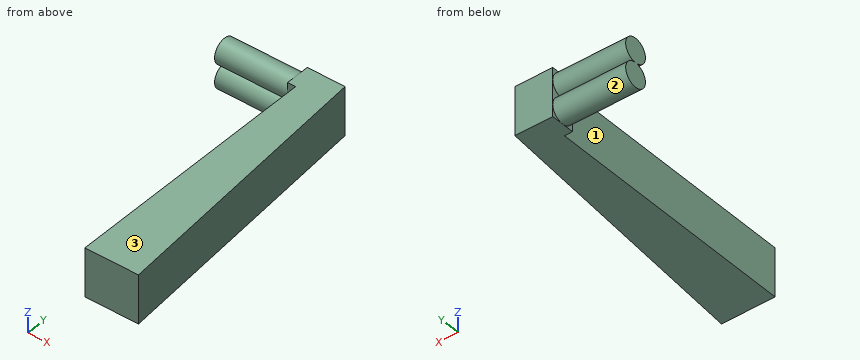
from build123d import *

# Parameters (mm, degrees)
ESTRUSIONE_ESTRUSIONE1_DEPTH      = 30
ESTRUSIONE_ESTRUSIONE1_DEPTH_BACK = 30
ESTRUSIONE_ESTRUSIONE2_DEPTH      = 100
SCHIZZO4_W                        = 60
SCHIZZO4_H                        = 30
ESTRUSIONE_ESTRUSIONE3_DEPTH      = 10


with BuildPart() as part:
    # Schizzo2 → Estrusione-Estrusione1 (new, two sides: drawn at the far end of the back side and taken through both)
    with BuildSketch(Plane.XY.offset(-ESTRUSIONE_ESTRUSIONE1_DEPTH_BACK)):
        Polygon((-15.384222889, 0), (50.78379402, 0), (21.335941259, 350), (-15.384222889, 350), align=None)
    extrude(amount=ESTRUSIONE_ESTRUSIONE1_DEPTH + ESTRUSIONE_ESTRUSIONE1_DEPTH_BACK)

    # Schizzo3 → Estrusione-Estrusione2 (add)
    with BuildSketch(Plane.ZY.offset(15.384222889)):
        with BuildLine():
            Line((-0.032724291, 335.990281697), (0.032724291, 335.990281697))
            ThreePointArc((0.032724291, 335.990281697), (29.999935115, 334.955880248), (0.027157826, 334.097782056))
            Line((0.027157826, 334.097782056), (-0.027157826, 334.097782056))
            ThreePointArc((-0.027157826, 334.097782056), (-29.999935115, 334.955880248), (-0.032724291, 335.990281697))
        make_face()
    extrude(amount=ESTRUSIONE_ESTRUSIONE2_DEPTH)

    # Schizzo4 → Estrusione-Estrusione3 (add)
    with BuildSketch(Plane.ZY.offset(15.384222889)):
        with Locations((0, 335)):
            Rectangle(SCHIZZO4_W, SCHIZZO4_H)
    extrude(amount=ESTRUSIONE_ESTRUSIONE3_DEPTH)


solid = part.part
For this review, take the finished solid that the model builds, in its own axes (mm). Face numbers are marked on the shaded views. Give positions to 0.01 mm unless a question says otherwise; leave off trailing zeros. Write each loop counter-clockwise with the first axis right and the second up, starting at its lowest first coordinate (ties: lowest second). Pieces come first, ordered by that corner, then holes. Notation, with made-up numbers: (23, -2.75) -> (54, -2.75) arc R30 cw to (54, 28.25) -> close; hole circle Ø3 at (-15.75, -34). An arc over 180 degrees is marked (long way). Use CSV: the item, a comma, the result in double quotes.
Q1. For P1, Ø12, axis at y = 210.5, z = -11.5, coming from the -X side; P2, Ø8, axis at x = -19.5, z = -5.5, coming from the -Y side; P3, Ø6, axis at x = -49.5, z = 9.5, coming from the -Y side, all flat-tipped, find the tip position at first contact; note any pin that passes through.
Conclusion:
P1,"x = -15.38"
P2,"y = 320"
P3,"y = 320.21"
Q2. Take a section at C-C, the plane y = 325. Write out the cut boundary in (x, z).
Conclusion:
outline,"(-115.38, -26.18) -> (-25.38, -26.18) -> (-25.38, -30) -> (23.44, -30) -> (23.44, 30) -> (-25.38, 30) -> (-25.38, 26.18) -> (-115.38, 26.18) -> (-115.38, 3.82) -> (-25.38, 3.82) -> (-25.38, -3.82) -> (-115.38, -3.82) -> close"
Q3. Take a section at A-A, the plane z = -23.5. Write out the cut boundary in (x, y), then the cut area to 3 significant figures.
Conclusion:
outline,"(-115.38, 322.64) -> (-25.38, 322.64) -> (-25.38, 320) -> (-15.38, 320) -> (-15.38, 0) -> (50.78, 0) -> (21.34, 350) -> (-25.38, 350) -> (-25.38, 347.36) -> (-115.38, 347.36) -> close"
area,"20,500 mm2"
Q4. Take a section at D-D, the plane y = 240. Write out the cut boundary in (x, z).
Conclusion:
outline,"(-15.38, -30) -> (30.59, -30) -> (30.59, 30) -> (-15.38, 30) -> close"
Q5. To check wall thickness, follow probe 1 along Z at (x, y) = (-41, 330); probe 2 along Y at (x, z) = (-66.5, 14.5); probe 3 along X at (y, z) = (183.5, 4.5). State the ranges of each line that lie inside material, in increasing order. Write a range as [from, to].
Conclusion:
probe 1,"[-29.14, -0.86], [0.86, 29.14]"
probe 2,"[320.01, 349.99]"
probe 3,"[-15.38, 35.34]"
Q6. Take a section at B-B, the plane x = -92. Write out the cut boundary in (y, z).
Conclusion:
outline,"(334.1, -0.03) arc R15 ccw (long way) to (335.99, -0.03) -> (335.99, 0.03) arc R15 ccw (long way) to (334.1, 0.03) -> close"
Q7. Mouldability with a two-part tool opening along Z and no side actions: class the marked faces 1, 2 and 3 as pulls with the +Z half, pulls with the -Z half, needs draft (parallel to the pull), parting line crosses it, or undercut.
Conclusion:
face 1,"needs draft"
face 2,"undercut"
face 3,"pulls with the +Z half"
